Input: part model. Units: mm. Frame: model coordinates. A direction names the side the tool comes from. Round coordinates to 2 decimals unless told otherwise and drop trailing zeros. Loops run counter-clockwise (first coordinate to the right, second up) from the corner with the lowest first, then second, coordinate; pieces in that order, holes last. Notation, with made-up numbers: (83.25, 43.5) -> (138.25, 43.5) arc R11 cw to (138.25, 58.5) -> close; hole circle Ø8 at (-13, 42). An arc over 180 degrees is marked (long way). Answer as a JSON object with one key per item and string values. Group by question number.
Item 1: Section query D-D on z = 1. Return loops of the section in (x, y), and give its area (3 significant figures).
Item 2: Material intervals for line 1 (Z direction, x = 0, y = 1.55); line 2 (X direction, y = 6, z = 7); line 3 (Y direction, x = 1.75, z = -4.5), sorted ascending. Write a range as [from, to].
Item 3: Draft query along X for faces 5 (the cylindrical face through (-3.499, 1.217, -16.515)), 6 (the flat face through (3.4, -2, 0)), 7 (the cylindrical face through (1.43, 4.73, -9.87)). Return one class per face: released by +X, released by -X, zero draft, split by the parting line, or undercut.
Item 4: Pin query (flat end, axial travel): pin 1 (2.5 mm diameter, centred on y = 5, z = -1.5, fed in from +X); pin 2 (1 mm diameter, centred on x = -0.5, z = 7.5, fed in from +Y); pin 3 (1.5 mm diameter, centred on y = 3.5, z = -7.5, fed in from -X); pin 4 (2.5 mm diameter, centred on x = 0, z = -14.15, fed in from -Y). Return the tip coordinate at first contact, or that it passes through.
Item 5: Section query C-C on x = 0. Return loops of the section in (y, z).
Item 6: Section query B-B on z = 14.15. Return loops of the section in (x, y), and give its area (3 significant figures).
Item 7: Set-up query: faces 1 (the flat face through (-0.3, 4.7, 9.7)), 2 (the flat face through (0, -2, -12)), 3 (the flat face through (-0.36, 4.67, -10.21)), 4 (the flat face through (0, -2, 12)). Return all of +Z, -Z, +X, -X, +Y, -Y with unobstructed straight access to the full face (end or side cutting, diameter ignored); none if empty.
Item 8: Section query A-A on y = 6. Return loops of the section in (x, z).
Autodesk Inventor part; units mm, degrees
ref_plane "YZ Plane" through (0, 0, 0) normal (1, 0, 0) x (0, 1, 0)
ref_plane "XZ Plane" through (0, 0, 0) normal (0, 1, 0) x (-1, 0, 0)
ref_plane "XY Plane" through (0, 0, 0) normal (0, 0, 1) x (1, 0, 0)
sketch "Sketch1" plane through (0, 0, 0) normal (0, 1, 0) x (-1, 0, 0)
  line L0 (3.8, 16.8) -> (-3.8, 16.8)
  line L1 (-3.8, 16.8) -> (-3.8, -16.8)
  line L2 (-3.8, -16.8) -> (3.8, -16.8)
  line L3 (3.8, -16.8) -> (3.8, 16.8)
  circle A0 centre (0, 14.15) radius 1.6
  circle A1 centre (0, -14.15) radius 1.6
  point P0 (0, 0)
  dimension "d0" = 33.6
  dimension "d1" = 7.6
  dimension "d2" = 16.8
  dimension "d3" = 3.8
  dimension "d4" = 3.2
  dimension "d5" = 3.2
  dimension "d6" = 28.3
  dimension "d7" = 14.15
extrude "Extrusion1" add sketch "Sketch1" along normal blind 2.4
fillet "Fillet1" radius 1 4 edges at (3.8, 1.2, 16.8) (-3.8, 1.2, 16.8) (3.8, 1.2, -16.8) (-3.8, 1.2, -16.8)
sketch "Sketch2" plane through (0, 2.4, 0) normal (0, 1, 0) x (1, 0, 0)
  line L0 (-2.35, -9.4813) -> (-2.35, 9.4813)
  line L1 (-2.35, 9.4813) -> (2.35, 11.2)
  line L2 (2.35, 11.2) -> (2.35, -11.2)
  line L3 (2.35, -11.2) -> (-2.35, -9.4813)
  line L4 (1.85, -10.4848) -> (-1.85, -9.1318)
  line L5 (-1.85, -9.1318) -> (-1.85, 9.1318)
  line L6 (-1.85, 9.1318) -> (1.85, 10.4848)
  line L7 (1.85, 10.4848) -> (1.85, -10.4848)
  point P0 (0, 0)
  dimension "d11" = 69.914
  dimension "d13" = 22.4
  dimension "d14" = 4.7
  dimension "d15" = 2.35
  dimension "d17" = 0.5
  dimension "d18" = 0.5
  dimension "d19" = 0.5
  dimension "d20" = 0.5
  dimension "d21" = 11.2
  dimension "d22" = 69.914
  dimension "d23" = 69.914
extrude "Extrusion2" add sketch "Sketch2" along normal blind 4.6
fillet "Fillet2" radius 1 8 edges at (-2.35, 4.7, -9.4813) (-2.35, 4.7, 9.4813) (2.35, 4.7, 11.2) (2.35, 4.7, -11.2) (-1.85, 4.7, -9.1318) (-1.85, 4.7, 9.1318) (1.85, 4.7, -10.4848) (1.85, 4.7, 10.4848)
sketch "Sketch3" plane through (0, 0, 0) normal (0, -1, 0) x (1, 0, 0)
  line L0 (3.4, 12) -> (-3.4, 12)
  line L1 (-3.4, 12) -> (-3.4, -12)
  line L2 (-3.4, -12) -> (3.4, -12)
  line L3 (3.4, -12) -> (3.4, 12)
  point P0 (0, 0)
  dimension "d27" = 24
  dimension "d28" = 6.8
  dimension "d29" = 12
  dimension "d30" = 3.4
extrude "Extrusion3" add sketch "Sketch3" along normal blind 3.5
equation "\"d5\" = d4"
equation "\"d22\" = d11"
properties part number "31pin male connector"
Solved:
{
 "1": {"outline": "(-3.8, 0) -> (-3.4, 0) -> (-3.4, -3.5) -> (3.4, -3.5) -> (3.4, 0) -> (3.8, 0) -> (3.8, 2.4) -> (2.35, 2.4) -> (2.35, 7) -> (1.85, 7) -> (1.85, 2.4) -> (-1.85, 2.4) -> (-1.85, 7) -> (-2.35, 7) -> (-2.35, 2.4) -> (-3.8, 2.4) -> close", "area": "46.6 mm²"},
 "2": {"line 1": "[-16.8, -15.75], [-12.55, 12.55], [15.75, 16.8]", "line 2": "[-2.35, -1.85], [1.85, 2.35]", "line 3": "[-3.5, 2.4]"},
 "3": {"face 5": "released by -X", "face 6": "released by +X", "face 7": "undercut"},
 "4": {"pin 1": "x = 2.35", "pin 2": "y = 2.4", "pin 3": "x = -2.35", "pin 4": "through"},
 "5": {"outline": "(-3.5, -12) -> (0, -12) -> (0, -12.55) -> (2.4, -12.55) -> (2.4, -10.34) -> (7, -10.34) -> (7, -9.81) -> (2.4, -9.81) -> (2.4, 9.81) -> (7, 9.81) -> (7, 10.34) -> (2.4, 10.34) -> (2.4, 12.55) -> (0, 12.55) -> (0, 12) -> (-3.5, 12) -> close; (0, -16.8) -> (2.4, -16.8) -> (2.4, -15.75) -> (0, -15.75) -> close; (0, 15.75) -> (2.4, 15.75) -> (2.4, 16.8) -> (0, 16.8) -> close"},
 "6": {"outline": "(-3.8, 0) -> (-1.6, 0) -> (-1.6, 2.4) -> (-3.8, 2.4) -> close; (1.6, 0) -> (3.8, 0) -> (3.8, 2.4) -> (1.6, 2.4) -> close", "area": "10.6 mm²"},
 "7": {"face 1": "+Y", "face 2": "-Z, +X, -X, -Y", "face 3": "-Z, -X, +Y", "face 4": "+Z, +X, -X, -Y"},
 "8": {"outline": "(-2.35, -8.78) arc R1 ccw to (-1.69, -9.72) -> (1.01, -10.71) arc R1 ccw to (2.35, -9.77) -> (2.35, 9.77) arc R1 ccw to (1.01, 10.71) -> (-1.69, 9.72) arc R1 ccw to (-2.35, 8.78) -> close; hole (-1.85, -8.43) arc R1 ccw to (-1.19, -9.37) -> (0.51, -9.99) arc R1 ccw to (1.85, -9.05) -> (1.85, 9.05) arc R1 ccw to (0.51, 9.99) -> (-1.19, 9.37) arc R1 ccw to (-1.85, 8.43) -> close"}
}
